Autodesk Inventor part; units mm, degrees
ref_plane "YZ Plane" through (0, 0, 0) normal (1, 0, 0) x (0, 1, 0)
ref_plane "XZ Plane" through (0, 0, 0) normal (0, 1, 0) x (-1, 0, 0)
ref_plane "XY Plane" through (0, 0, 0) normal (0, 0, 1) x (1, 0, 0)
ref_plane "Płaszczyzna konstrukcyjna1" through (0, 0, 0) normal (0, 0, 1) x (1, 0, 0)
sketch "Szkic1" plane through (0, 0, 0) normal (0, 0, 1) x (1, 0, 0)
  circle A0 centre (-10, 0) radius 10
  circle A1 centre (-10, 0) radius 15
  circle A2 centre (-10, 0) radius 10
  circle A3 centre (-10, 0) radius 8
  circle A4 centre (-10, 0) radius 8
  circle A5 centre (-10, 0) radius 2
  point P0 (0, 0)
  dimension "d0" = 4
extrude "Wyciągnięcie proste1" add sketch "Szkic1" against normal blind 30 contours A3
sketch "Szkic2" plane through (-10, 0, 0) normal (0, 0, 1) x (1, 0, 0)
  circle A0 centre (0, 0) radius 8
  circle A1 centre (0, 0) radius 2
  circle A2 centre (0, 0) radius 2
  circle A3 centre (0, 0) radius 2
  circle A4 centre (0, 0) radius 14
  circle A5 centre (0, 0) radius 14
  point P0 (10, 0)
extrude "Wyciągnięcie proste2" add sketch "Szkic2" along normal blind 30 contours A0 | A4
sketch "Szkic3" plane through (-10, 0, 30) normal (0, 0, 1) x (1, 0, 0)
  circle A0 centre (0, 0) radius 2
  circle A1 centre (0, 0) radius 10
  point P0 (10, 0)
  dimension "d5" = 20
extrude "Wyciągnięcie proste3" cut sketch "Szkic3" against normal blind 10
sketch "Szkic4" plane through (-10, 0, 20) normal (0, 0, 1) x (1, 0, 0)
  circle A0 centre (0, 0) radius 5
  point P0 (10, 0)
  dimension "d8" = 10
extrude "Wyciągnięcie proste4" cut sketch "Szkic4" against normal blind 20
chamfer "Faza1" distance 1 angle 45 5 edges at (-20, 0, 30) (-15, 0, 20) (-24, 0, 30) (-24, 0, 0) (-18, 0, -30)
properties part number "korek" material "Polietylen, o małej gęstości"
Build history of the part. All positions in model axes, mm. A direction names the side the tool comes from. Give positions to 0.01 mm unless a question says otherwise; leave off trailing zeros. Order: outer loops, then holes, each group sorted by start corner. A loop starts at its lowest first (then second) coordinate and runs counter-clockwise, first axis right, second up. Notation, with made-up numbers: M 52,-3 L 67,-3 A30 cw 67,28 Z; hole C 74,62.5 d2. An arc over 180 degrees is marked long. Put each result on its own line as item: value.
Item 1: Cut at D-D on z = -10. Write the cut outline in (x, y), then the cut area to 3 significant figures.
Results are:
outline: C -10,0 d16; hole C -10,0 d4
area: 188 mm2
Item 2: Pull direction Y, two halves, no side cores. Call faces 4 (the face through (3.35, -4.21, 14.8)), 5 (the face through (-16, -6, 0)), 6 (the face through (-10, -7, 20)): +Y half, -Y half, draft (parallel to the pull), parting line (faces both ways), or undercut.
Results are:
face 4: parting line
face 5: draft
face 6: undercut
Item 3: Cut at C-C on z = 8. Write the cut outline in (x, y).
Results are:
outline: C -10,0 d28; hole C -10,0 d10
Item 4: Drop flat-ended pins along their axis: pin 1 Ø2 at (y, z) = (-2, -21.5) entering from +X; pin 2 Ø12 at (x, y) = (-10, -7.5) entering from -Z; pin 3 Ø8 at (x, z) = (-4, 5) entering from -Y; pin 4 Ø8 at (y, z) = (3, -22) entering from +X. Give the stop position or say it passes through.
Results are:
pin 1: x = -2.06
pin 2: z = -30
pin 3: y = -13.86
pin 4: x = -2
Item 5: Which spindle directions (+Z, -Z, +X, -X, +Y, -Y) get a long thin tool onto all of the face, cutting with end or side? Do faces 1 (the face through (-11.73, -7.81, -14.3)), 2 (the face through (-10.1, -2.2, 0)), 3 (the face through (-11.6, -1.2, -14.8)). Say none if no direction does.
Results are:
face 1: -Z
face 2: +Z
face 3: +Z, -Z
Item 6: Wall check: probe 1 along X at (y, z) = (-0.25, 27); probe 2 along Y at (x, z) = (-10, 22); probe 3 along Y at (x, z) = (-10, -16). Give the ranges that are in metal, low to high.
Results are:
probe 1: -24 to -20, 0 to 4
probe 2: -14 to -10, 10 to 14
probe 3: -8 to -2, 2 to 8
